Autodesk Inventor part; units mm, degrees
ref_plane "YZ Plane" through (0, 0, 0) normal (1, 0, 0) x (0, 1, 0)
ref_plane "XZ Plane" through (0, 0, 0) normal (0, 1, 0) x (-1, 0, 0)
ref_plane "XY Plane" through (0, 0, 0) normal (0, 0, 1) x (1, 0, 0)
sketch "Sketch1" plane through (0, 0, 0) normal (0, 0, 1) x (1, 0, 0)
  line L0 (0, 0) -> (18.6, 0)
  line L1 (18.6, 0) -> (18.6, 61.5)
  line L2 (18.6, 61.5) -> (0, 61.5)
  line L3 (0, 61.5) -> (0, 0)
  circle A0 centre (8, 10) radius 2.7436
  circle A1 centre (8, 51) radius 2.7436
  dimension "d0" = 61.5
  dimension "d1" = 18.6
  dimension "d2" = 10
  dimension "d3" = 8
  dimension "d4" = 8
  dimension "d5" = 10.5
extrude "Extrusion1" add sketch "Sketch1" along normal blind 3
properties part number "pulley_tab_left_B"
Check sheet for the modelled part. Datum: model origin and axes. Units: mm. Give positions to 0.01 mm unless a question says otherwise; leave off trailing zeros. Loops run counter-clockwise (first coordinate to the right, second up) from the corner with the lowest first, then second, coordinate; pieces in that order, holes last. Notation, with made-up numbers: M -2,28.25 L 31,28.25 A28 ccw 31,52.25 Z; hole C 88.5,84.5 d8. An arc over 180 degrees is marked long. Answer as a JSON object with one key per item and string values. Group by question number.
Q1. Cross-section at B-B on x = 8. Record the cut outline in (y, z).
Q2. Cross-section at C-C on z = 0.5. Record the cut outline in (x, y), then the cut area to 3 significant figures.
Q3. Cross-section at A-A on y = 51. Record the cut outline in (x, z), then the cut area to 3 significant figures.
Q4. Material ranges on line 1 along Y through (x, z) = (8, 0.75); line 2 along X through (y, z) = (11, 1.45); line 3 along X through (y, z) = (12.5, 1.9), recorded low to high. Write a range as [from, to].
Q5. Release check for a two-part mould opening along X. For faces 1 (the flat face through (18.6, 30, 1)), 2 (the cylindrical face through (5.26, 9.88, 1.48)), 3 (the flat face through (0, 31, 1)) record: released by +X, released by -X, zero draft, split by the parting line, or undercut.
Evaluation:
{
 "1": {"outline": "M 0,0 L 7.26,0 L 7.26,3 L 0,3 Z; M 12.74,0 L 48.26,0 L 48.26,3 L 12.74,3 Z; M 53.74,0 L 61.5,0 L 61.5,3 L 53.74,3 Z"},
 "2": {"outline": "M 0,0 L 18.6,0 L 18.6,61.5 L 0,61.5 Z; hole C 8,10 d5.49; hole C 8,51 d5.49", "area": "1,100 mm2"},
 "3": {"outline": "M 0,0 L 5.26,0 L 5.26,3 L 0,3 Z; M 10.74,0 L 18.6,0 L 18.6,3 L 10.74,3 Z", "area": "39.3 mm2"},
 "4": {"line 1": "y = [0, 7.26], [12.74, 48.26], [53.74, 61.5]", "line 2": "x = [0, 5.45], [10.55, 18.6]", "line 3": "x = [0, 6.87], [9.13, 18.6]"},
 "5": {"face 1": "released by +X", "face 2": "undercut", "face 3": "released by -X"}
}
